from build123d import *

# Parameters (mm, degrees)
SKETCH_1_W      = 30
SKETCH_1_H      = 30
EXTRUDE_1_DEPTH = 40
SKETCH_2_W      = 30
SKETCH_2_H      = 10.165772452
EXTRUDE_2_DEPTH = 60
SKETCH_3_R      = 12
EXTRUDE_3_DEPTH = 5
SKETCH_4_R      = 9
EXTRUDE_4_DEPTH = 5


with BuildPart() as part:
    # Эскиз1 → Бобышка-Вытянуть1 (new body)
    with BuildSketch(Plane(origin=(0, 0, 0), x_dir=(0, 0, -1), z_dir=(1, 0, 0))):
        with Locations((-24.657846844, 7.360988518)):
            Rectangle(SKETCH_1_W, SKETCH_1_H)
    extrude(amount=EXTRUDE_1_DEPTH)

    # Эскиз2 → Бобышка-Вытянуть2 (add)
    with BuildSketch(Plane(origin=(40, 0, 0), x_dir=(0, 0, -1), z_dir=(1, 0, 0))):
        with Locations((-24.657846844, 17.278102292)):
            Rectangle(SKETCH_2_W, SKETCH_2_H)
    extrude(amount=EXTRUDE_2_DEPTH)

    # Эскиз3 → Бобышка-Вытянуть3 (add)
    with BuildSketch(Plane.XZ.offset(-12.195216066)):
        with Locations(Location((85.620234383, 24.657846844, 0), (0, 0, 90))):
            Circle(SKETCH_3_R)
    extrude(amount=EXTRUDE_3_DEPTH)

    # Эскиз4 → Бобышка-Вытянуть4 (add)
    with BuildSketch(Plane.XZ.offset(-7.195216066)):
        with Locations(Location((85.620234383, 24.657846844, 0), (0, 0, 270))):
            Circle(SKETCH_4_R)
    extrude(amount=EXTRUDE_4_DEPTH)

    # Эскиз13 → Цековка для  болта с шестигранной головкой M51 (revolve, cut)
    with BuildSketch(Plane(origin=(40, 2.482471753, 24.681970174), x_dir=(0, 0, -1), z_dir=(0, 1, 0))):
        Polygon((0, 0), (0, 40), (2.75, 40), (2.75, 3.5), (6.119, 3.5), (6.119, 0.025), (6.144, 0), align=None)
    revolve(axis=Axis((46.35, 2.482471753, 24.681970174), (-1, 0, 0)), mode=Mode.SUBTRACT)


solid = part.part
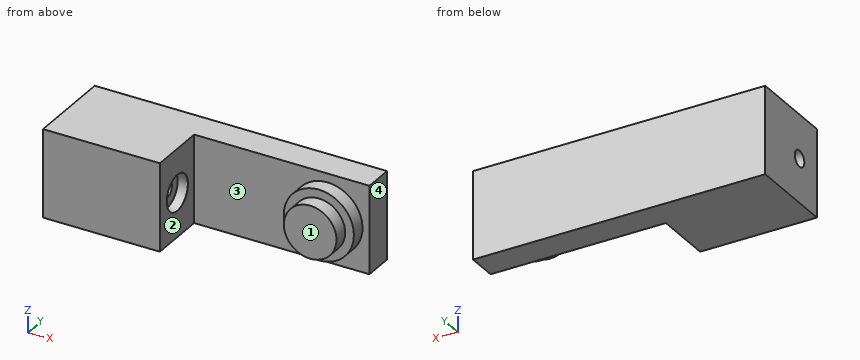
Geometry check sheet. Reference: the model listing, model coordinates, mm. Face numbers are marked on the shaded views. Round coordinates to 2 decimals unless told otherwise and drop trailing zeros. Order: outer loops, then holes, each group sorted by start corner. A loop starts at its lowest first (then second) coordinate and runs counter-clockwise, first axis right, second up. Notation, with made-up numbers: M 65,79 L 74,79 A22 ccw 74,113 Z; hole C 57.25,36.5 d4. An arc over 180 degrees is marked long. Answer in a Markdown table with one row per item.
(1) Sectioned sample at C-C, the plane x = 87.5. Record the cut outline in (y, z), and give its area (3 significant figures).
Responses:
| item | result |
|---|---|
| outline | M 2.2,15.86 L 7.2,15.86 L 7.2,12.81 L 12.2,12.81 L 12.2,9.66 L 22.36,9.66 L 22.36,39.66 L 12.2,39.66 L 12.2,36.51 L 7.2,36.51 L 7.2,33.46 L 2.2,33.46 Z |
| area | 512 mm² |
(2) Go/stop test with flat-tipped pins: P1, Ø6, axis at y = 3, z = 24, coming from the +X side; P2, Ø2, axis at y = 15, z = 23.5, coming from the -X side; P3, Ø10, axis at y = 3, z = 21.5, coming from the +X side. Record where each tip stops, or that it passes through.
Responses:
| item | result |
|---|---|
| P1 | stops at x = 94.62 |
| P2 | stops at x = 0 |
| P3 | stops at x = 97.61 |
(3) Sectioned sample at B-B, the plane x = 62. Record the cut outline in (y, z), and give its area (3 significant figures).
Responses:
| item | result |
|---|---|
| outline | M 12.2,9.66 L 22.36,9.66 L 22.36,39.66 L 12.2,39.66 Z |
| area | 305 mm² |
(4) Scan lines: probe 1 along Z at (x, y) = (5, 2.75); probe 2 along Y at (x, z) = (85, 22.5); probe 3 along Y at (x, z) = (59, 20.5). Record each from-to range of solid material in increasing order. Write a range as from..to.
Responses:
| item | result |
|---|---|
| probe 1 | z = 9.66..21.95, 27.42..39.66 |
| probe 2 | y = 2.2..22.36 |
| probe 3 | y = 12.2..22.36 |
(5) Sectioned sample at A-A, the plane x = 6.5. Record the cut outline in (y, z), and give its area (3 significant figures).
Responses:
| item | result |
|---|---|
| outline | M -7.64,9.66 L 22.36,9.66 L 22.36,39.66 L -7.64,39.66 Z; hole C 2.48,24.68 d5.5 |
| area | 876 mm² |
(6) Draft check along X on the marked faces 1, 2, 3 and 4. Enter one of: released by +X, released by -X, zero draft, split by the parting line, or undercut.
Responses:
| item | result |
|---|---|
| face 1 | zero draft |
| face 2 | undercut |
| face 3 | undercut |
| face 4 | released by +X |
